```python
from build123d import *

# Parameters (mm, degrees)
SKETCH1_W                              = 228
SKETCH1_H                              = 25
BOSS_EXTRUDE1_DEPTH                    = 60
SKETCH3_W                              = 12.5
SKETCH3_H                              = 12.5
CUT_EXTRUDE2_DEPTH                     = 10
LPATTERN1_COUNT                        = 2
LPATTERN1_PITCH                        = 102.5
SKETCH7_R                              = 7.5
BOSS_EXTRUDE4_DEPTH                    = 3
BOSS_EXTRUDE4_DRAFT                    = 20
BOSS_EXTRUDE4_PROFILE_2_DEPTH          = 3
BOSS_EXTRUDE4_PROFILE_2_DRAFT          = 20
BOSS_EXTRUDE4_PROFILE_3_DEPTH          = 3
BOSS_EXTRUDE4_PROFILE_3_DRAFT          = 20
BOSS_EXTRUDE4_PROFILE_4_DEPTH          = 3
BOSS_EXTRUDE4_PROFILE_4_DRAFT          = 20
M3X0_5_TAPPED_HOLE1_D                  = 2.5
M3X0_5_TAPPED_HOLE1_DEPTH              = 5
M3X0_5_TAPPED_HOLE1_TIP                = 0.751075774
SKETCH12_W                             = 35
SKETCH12_H                             = 25
CUT_EXTRUDE3_DEPTH                     = 15
SKETCH6_R                              = 7
CUT_EXTRUDE4_DEPTH                     = 10
F_4_5_4_5_DRILL_BIT_FOR_PEM_NUTS_D     = 4.5
F_4_5_4_5_DRILL_BIT_FOR_PEM_NUTS_DEPTH = 5
F_4_5_4_5_DRILL_BIT_FOR_PEM_NUTS_TIP   = 1.351936393


with BuildPart() as part:
    # Sketch1 → Boss-Extrude1 (new, symmetric)
    with BuildSketch(Plane.XY):
        Rectangle(SKETCH1_W, SKETCH1_H)
    extrude(amount=BOSS_EXTRUDE1_DEPTH, both=True)

    # Sketch3 → Cut-Extrude2 (cut)
    with BuildSketch(Plane.XY.offset(60)):
        with Locations((82.75, -1.25)):
            Rectangle(SKETCH3_W, SKETCH3_H)
        with Locations((97.75, -1.25)):
            Rectangle(SKETCH3_W, SKETCH3_H)
        with Locations((67.75, -1.25)):
            Rectangle(SKETCH3_W, SKETCH3_H)
        with Locations((52.75, -1.25)):
            Rectangle(SKETCH3_W, SKETCH3_H)
        with Locations((37.75, -1.25)):
            Rectangle(SKETCH3_W, SKETCH3_H)
    cut_extrude2 = extrude(amount=-CUT_EXTRUDE2_DEPTH, mode=Mode.SUBTRACT)

    # LPattern1: Cut-Extrude2 ×2
    with Locations(*[(-i * LPATTERN1_PITCH, 0, 0) for i in range(1, LPATTERN1_COUNT)]):
        add(cut_extrude2, mode=Mode.SUBTRACT)


with BuildPart() as boss_extrude4_tool:
    # Sketch7 → Boss-Extrude4 (with draft: the straight prism first)
    with BuildSketch(Plane.XZ.offset(12.5)):
        with Locations((-84, -25)):
            Circle(SKETCH7_R)
    extrude(amount=BOSS_EXTRUDE4_DEPTH)
    # Boss-Extrude4: the draft: its side faces are tilted about the plane it starts from
    boss_extrude4_sides = [boss_extrude4_tool.faces().sort_by_distance(p)[0] for p in [
        (-91.5, -14, -25),
    ]]
    draft(boss_extrude4_sides, Plane.XZ.offset(12.5), BOSS_EXTRUDE4_DRAFT)


with BuildPart() as part_1:
    add(part.part)

    # Boss-Extrude4: add boss_extrude4_tool
    add(boss_extrude4_tool.part)


with BuildPart() as boss_extrude4_profile_2_tool:
    # Sketch7 → Boss-Extrude4 profile 2 (with draft: the straight prism first)
    with BuildSketch(Plane.XZ.offset(12.5)):
        with Locations((-84, 40)):
            Circle(SKETCH7_R)
    extrude(amount=BOSS_EXTRUDE4_PROFILE_2_DEPTH)
    # Boss-Extrude4 profile 2: the draft: its side faces are tilted about the plane it starts from
    boss_extrude4_profile_2_sides = [boss_extrude4_profile_2_tool.faces().sort_by_distance(p)[0] for p in [
        (-91.5, -14, 40),
    ]]
    draft(boss_extrude4_profile_2_sides, Plane.XZ.offset(12.5), BOSS_EXTRUDE4_PROFILE_2_DRAFT)


with BuildPart() as part_2:
    add(part_1.part)

    # Boss-Extrude4 profile 2: add boss_extrude4_profile_2_tool
    add(boss_extrude4_profile_2_tool.part)


with BuildPart() as boss_extrude4_profile_3_tool:
    # Sketch7 → Boss-Extrude4 profile 3 (with draft: the straight prism first)
    with BuildSketch(Plane.XZ.offset(12.5)):
        with Locations((84, 40)):
            Circle(SKETCH7_R)
    extrude(amount=BOSS_EXTRUDE4_PROFILE_3_DEPTH)
    # Boss-Extrude4 profile 3: the draft: its side faces are tilted about the plane it starts from
    boss_extrude4_profile_3_sides = [boss_extrude4_profile_3_tool.faces().sort_by_distance(p)[0] for p in [
        (76.5, -14, 40),
    ]]
    draft(boss_extrude4_profile_3_sides, Plane.XZ.offset(12.5), BOSS_EXTRUDE4_PROFILE_3_DRAFT)


with BuildPart() as part_3:
    add(part_2.part)

    # Boss-Extrude4 profile 3: add boss_extrude4_profile_3_tool
    add(boss_extrude4_profile_3_tool.part)


with BuildPart() as boss_extrude4_profile_4_tool:
    # Sketch7 → Boss-Extrude4 profile 4 (with draft: the straight prism first)
    with BuildSketch(Plane.XZ.offset(12.5)):
        with Locations((84, -25)):
            Circle(SKETCH7_R)
    extrude(amount=BOSS_EXTRUDE4_PROFILE_4_DEPTH)
    # Boss-Extrude4 profile 4: the draft: its side faces are tilted about the plane it starts from
    boss_extrude4_profile_4_sides = [boss_extrude4_profile_4_tool.faces().sort_by_distance(p)[0] for p in [
        (76.5, -14, -25),
    ]]
    draft(boss_extrude4_profile_4_sides, Plane.XZ.offset(12.5), BOSS_EXTRUDE4_PROFILE_4_DRAFT)


with BuildPart() as part_4:
    add(part_3.part)

    # Boss-Extrude4 profile 4: add boss_extrude4_profile_4_tool
    add(boss_extrude4_profile_4_tool.part)

    # M3x0.5 Tapped Hole1
    with Locations(Plane(origin=(0, -12.5, 0), x_dir=(-1, 0, 0), z_dir=(0, -1, 0))):
        with Locations((105.75, -25), (-105.75, -25)):
            Hole(M3X0_5_TAPPED_HOLE1_D / 2, depth=M3X0_5_TAPPED_HOLE1_DEPTH)
            with Locations((0, 0, -(M3X0_5_TAPPED_HOLE1_DEPTH + M3X0_5_TAPPED_HOLE1_TIP / 2))):  # 118° drill point
                Cone(0, M3X0_5_TAPPED_HOLE1_D / 2, M3X0_5_TAPPED_HOLE1_TIP, mode=Mode.SUBTRACT)

    # Sketch12 → Cut-Extrude3 (cut)
    with BuildSketch(Plane.XZ.offset(12.5)):
        with Locations((-76.5, -47.5)):
            Rectangle(SKETCH12_W, SKETCH12_H)
    extrude(amount=-CUT_EXTRUDE3_DEPTH, mode=Mode.SUBTRACT)

    # Sketch6 → Cut-Extrude4 (cut)
    with BuildSketch(Plane(origin=(0, 0, -60), x_dir=(-1, 0, 0), z_dir=(0, 0, -1))):
        with Locations((-103, 0)):
            Circle(SKETCH6_R)
        with Locations((-29, 0)):
            Circle(SKETCH6_R)
        with Locations((29, 0)):
            Circle(SKETCH6_R)
        with Locations((103, 0)):
            Circle(SKETCH6_R)
    extrude(amount=-CUT_EXTRUDE4_DEPTH, mode=Mode.SUBTRACT)

    # Ø4.5 (4.5) Drill Bit for PEM Nuts
    with Locations(Plane(origin=(0, 12.5, 0), x_dir=(1, 0, 0), z_dir=(0, 1, 0))):
        with Locations((-4, -51.5), (-75.5, 23.2), (103.5, 23.5)):
            Hole(F_4_5_4_5_DRILL_BIT_FOR_PEM_NUTS_D / 2, depth=F_4_5_4_5_DRILL_BIT_FOR_PEM_NUTS_DEPTH)
            with Locations((0, 0, -(F_4_5_4_5_DRILL_BIT_FOR_PEM_NUTS_DEPTH + F_4_5_4_5_DRILL_BIT_FOR_PEM_NUTS_TIP / 2))):  # 118° drill point
                Cone(0, F_4_5_4_5_DRILL_BIT_FOR_PEM_NUTS_D / 2, F_4_5_4_5_DRILL_BIT_FOR_PEM_NUTS_TIP, mode=Mode.SUBTRACT)


solid = part_4.part
```
Part model, mm, in its own coordinate system. A direction names the side the tool comes from. Round coordinates to 2 decimals unless told otherwise and drop trailing zeros. Order: outer loops, then holes, each group sorted by start corner. A loop starts at its lowest first (then second) coordinate and runs counter-clockwise, first axis right, second up. Notation, with made-up numbers: M -12,60 L -1,60 A6 cw -1,64 Z; hole C 77,53 d6. An arc over 180 degrees is marked long. Put each result on its own line as item: value. Start each with the question number.
1. Drop flat-ended pins along their axis: pin 1 (10 mm diameter, centred on x = -17, y = -1.5, fed in from +Z); pin 2 (3 mm diameter, centred on x = 65.5, z = 53.5, fed in from -Y); pin 3 (6 mm diameter, centred on x = 38.5, y = 0.5, fed in from +Z). Give the stop position or say it passes through.
2. Tool access for faces 1 (the face through (114, 0, 1)), 2 (the face through (-50, -1, 50)), 3 (the face through (22.323, 2.103, -55.07)): list every direction of +Z, -Z, +X, -X, +Y, -Y with a clear straight run to the whole face (end or side of a thin tool).
3. Slice it at D-D on z = -2. List the corners of the cut face in (x, y), then the cut area to 3 significant figures.
4. Slice it at B-B on z = 40. List the corners of the cut face in (x, y).
5. Two-plate mould, pull along Z, no slides. Class faces 4 (the face through (-77.823, -15.312, -23.055)), 5 (the face through (-5, -1, 50)), 6 (the face through (61.5, -1, 55)): +Z half, -Z half, draft (parallel to the pull), parting line (faces both ways), or undercut.
6. Slice it at C-C on x = 84. List the corners of the cut face in (y, z).
7. Drill centre lines: probe 1 along X at (y, z) = (-9.95, 25); probe 2 along Y at (x, z) = (-29, -53); probe 3 along Z at (x, y) = (-4, 8.8). Where is each one in solid material? Low to high. Write a range as [from, to].
8. Slice it at A-A on x = 29. List the corners of the cut face in (y, z).
Findings:
1. pin 1: z = 60
1. pin 2: y = -12.5
1. pin 3: z = 50
2. face 1: +Z, -Z, +X, +Y, -Y
2. face 2: +Z
2. face 3: -Z
3. outline: M -114,-12.5 L 114,-12.5 L 114,12.5 L -114,12.5 Z
3. area: 5,700 mm2
4. outline: M -114,-12.5 L -91.5,-12.5 L -90.41,-15.5 L -77.59,-15.5 L -76.5,-12.5 L 76.5,-12.5 L 77.59,-15.5 L 90.41,-15.5 L 91.5,-12.5 L 114,-12.5 L 114,12.5 L -114,12.5 Z
5. face 4: undercut
5. face 5: +Z half
5. face 6: draft
6. outline: M -15.5,-31.41 L -12.5,-32.5 L -12.5,-60 L 12.5,-60 L 12.5,60 L 5,60 L 5,50 L -7.5,50 L -7.5,60 L -12.5,60 L -12.5,47.5 L -15.5,46.41 L -15.5,33.59 L -12.5,32.5 L -12.5,-17.5 L -15.5,-18.59 Z
7. probe 1: [-114, -107], [-104.5, 104.5], [107, 114]
7. probe 2: [-12.5, -7], [7, 12.5]
7. probe 3: [-60, 49.25], [53.75, 60]
8. outline: M -12.5,-60 L -7,-60 L -7,-50 L 7,-50 L 7,-60 L 12.5,-60 L 12.5,60 L -12.5,60 Z
